from build123d import *

# Parameters (mm, degrees)
SKETCH1_R                 = 2.5
SKETCH1_R_2               = 3
BOSS_EXTRUDE1_DEPTH       = 6.35
SKETCH2_R                 = 1
POTENTIOMETER_HOLES_DEPTH = 39.839927909


with BuildPart() as part:
    # Sketch1 → Boss-Extrude1 (new, symmetric)
    with BuildSketch(Plane(origin=(0, 0, 0), x_dir=(1, 0, 0), z_dir=(0, 1, 0))):
        with BuildLine():
            Line((-21.150952157, 4.29136197), (-6.150952157, 25.79136197))
            ThreePointArc((-6.150952157, 25.79136197), (0, 29), (6.150952157, 25.79136197))
            Line((6.150952157, 25.79136197), (21.150952157, 4.29136197))
            ThreePointArc((21.150952157, 4.29136197), (22.5, 0), (21.150952157, -4.29136197))
            Line((21.150952157, -4.29136197), (6.150952157, -25.79136197))
            ThreePointArc((6.150952157, -25.79136197), (0, -29), (-6.150952157, -25.79136197))
            Line((-6.150952157, -25.79136197), (-21.150952157, -4.29136197))
            ThreePointArc((-21.150952157, -4.29136197), (-22.5, 0), (-21.150952157, 4.29136197))
        make_face()
        with Locations(Location((0, 21.5, 0), (0, 0, 270))):
            Circle(SKETCH1_R, mode=Mode.SUBTRACT)
        with Locations(Location((0, -21.5, 0), (0, 0, 270))):
            Circle(SKETCH1_R, mode=Mode.SUBTRACT)
        with Locations(Location((-10, 0, 0), (0, 0, 270))):
            Circle(SKETCH1_R_2, mode=Mode.SUBTRACT)
        with Locations(Location((10, 0, 0), (0, 0, 270))):
            Circle(SKETCH1_R_2, mode=Mode.SUBTRACT)
    extrude(amount=BOSS_EXTRUDE1_DEPTH, both=True)

    # Sketch2 → Potentiometer Holes (cut, through all)
    with BuildSketch(Plane(origin=(0, 6.35, 0), x_dir=(1, 0, 0), z_dir=(0, 1, 0))):
        with Locations(Location((-17.5, 0, 0), (0, 0, 270))):
            Circle(SKETCH2_R)
        with Locations(Location((17.5, 0, 0), (0, 0, 270))):
            Circle(SKETCH2_R)
        with Locations(Location((0, 0, 0), (0, 0, 270))):
            Circle(SKETCH2_R)
    extrude(amount=-POTENTIOMETER_HOLES_DEPTH, mode=Mode.SUBTRACT)


solid = part.part
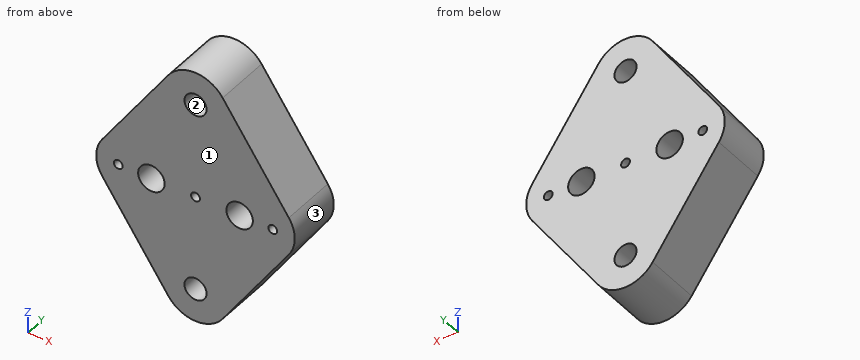
Could you check a few things on this model? Use its own coordinates, in mm. Face numbers are marked on the shaded views. Give positions to 0.01 mm unless a question says otherwise; leave off trailing zeros. Loops run counter-clockwise (first coordinate to the right, second up) from the corner with the lowest first, then second, coordinate; pieces in that order, holes last. Notation, with made-up numbers: (-8.75, 4) -> (21.25, 4) arc R5 ccw to (21.25, 13) -> close; hole circle Ø6 at (84.25, -31.5). An arc over 180 degrees is marked (long way). Return JSON: item names as keys, results as strings.
Item 1: If we section it at B-B on z = 0: List the corners of the cut face in (x, y) for me, plus the area to 3 significant figures.
Geometry results:
{"outline": "(-22.5, -6.35) -> (-18.5, -6.35) -> (-18.5, 6.35) -> (-22.5, 6.35) -> close; (-16.5, -6.35) -> (-13, -6.35) -> (-13, 6.35) -> (-16.5, 6.35) -> close; (-7, -6.35) -> (-1, -6.35) -> (-1, 6.35) -> (-7, 6.35) -> close; (1, -6.35) -> (7, -6.35) -> (7, 6.35) -> (1, 6.35) -> close; (13, -6.35) -> (16.5, -6.35) -> (16.5, 6.35) -> (13, 6.35) -> close; (18.5, -6.35) -> (22.5, -6.35) -> (22.5, 6.35) -> (18.5, 6.35) -> close", "area": "343 mm²"}
Item 2: I'm going to push flat-ended pins straight in: pin 1 (2 mm diameter, centred on y = 2, z = -9, fed in from +X); pin 2 (2 mm diameter, centred on y = 5, z = 17.5, fed in from -X); pin 3 (1.2 mm diameter, centred on x = -17.5, z = 0, fed in from +Y); pin 4 (1 mm diameter, centred on y = 3.5, z = -19.5, fed in from -X). Where does each tip first touch, or does it pass through?
Geometry results:
{"pin 1": "stops at x = 18.56", "pin 2": "stops at x = -12.63", "pin 3": "passes through", "pin 4": "stops at x = -10.89"}
Item 3: I need wall thicknesses on L1, parallel to X at y = 3, z = 0; L2, parallel to Z at x = -2, y = 2.75; L3, parallel to X at y = -0.25, z = 21.5. Which ranges of each line are inside material? Lowest first, please. Write a range as from..to.
Geometry results:
{"L1": "x = -22.5..-18.5, -16.5..-13, -7..-1, 1..7, 13..16.5, 18.5..22.5", "L2": "z = -28.73..-23, -20..20, 23..28.73", "L3": "x = -9.14..-2.5, 2.5..9.14"}
Item 4: If we section it at C-C on x = 0: List the corners of the cut face in (y, z) for me, plus the area to 3 significant figures.
Geometry results:
{"outline": "(-6.35, -29) -> (6.35, -29) -> (6.35, -24) -> (-6.35, -24) -> close; (-6.35, -19) -> (6.35, -19) -> (6.35, -1) -> (-6.35, -1) -> close; (-6.35, 1) -> (6.35, 1) -> (6.35, 19) -> (-6.35, 19) -> close; (-6.35, 24) -> (6.35, 24) -> (6.35, 29) -> (-6.35, 29) -> close", "area": "584 mm²"}
Item 5: If we section it at A-A on y = -0.25: List the corners of the cut face in (x, z) for me.
Geometry results:
{"outline": "(-21.15, -4.29) -> (-6.15, -25.79) arc R7.5 ccw to (6.15, -25.79) -> (21.15, -4.29) arc R7.5 ccw to (21.15, 4.29) -> (6.15, 25.79) arc R7.5 ccw to (-6.15, 25.79) -> (-21.15, 4.29) arc R7.5 ccw to start; hole circle Ø2 at (-17.5, 0); hole circle Ø6 at (-10, 0); hole circle Ø5 at (0, -21.5); hole circle Ø5 at (0, 21.5); hole circle Ø2 at (0, 0); hole circle Ø6 at (10, 0); hole circle Ø2 at (17.5, 0)"}
Item 6: If we section it at D-D on x = 10: List the corners of the cut face in (y, z) for me, plus the area to 3 significant figures.
Geometry results:
{"outline": "(-6.35, -20.27) -> (6.35, -20.27) -> (6.35, -3) -> (-6.35, -3) -> close; (-6.35, 3) -> (6.35, 3) -> (6.35, 20.27) -> (-6.35, 20.27) -> close", "area": "439 mm²"}
Item 7: We'd pull the mould along Z, two halves only. Please class the marked faces 1, 2 and 3: +Z half, -Z half, draft (parallel to the pull), parting line (faces both ways), or undercut.
Geometry results:
{"face 1": "draft", "face 2": "undercut", "face 3": "parting line"}
